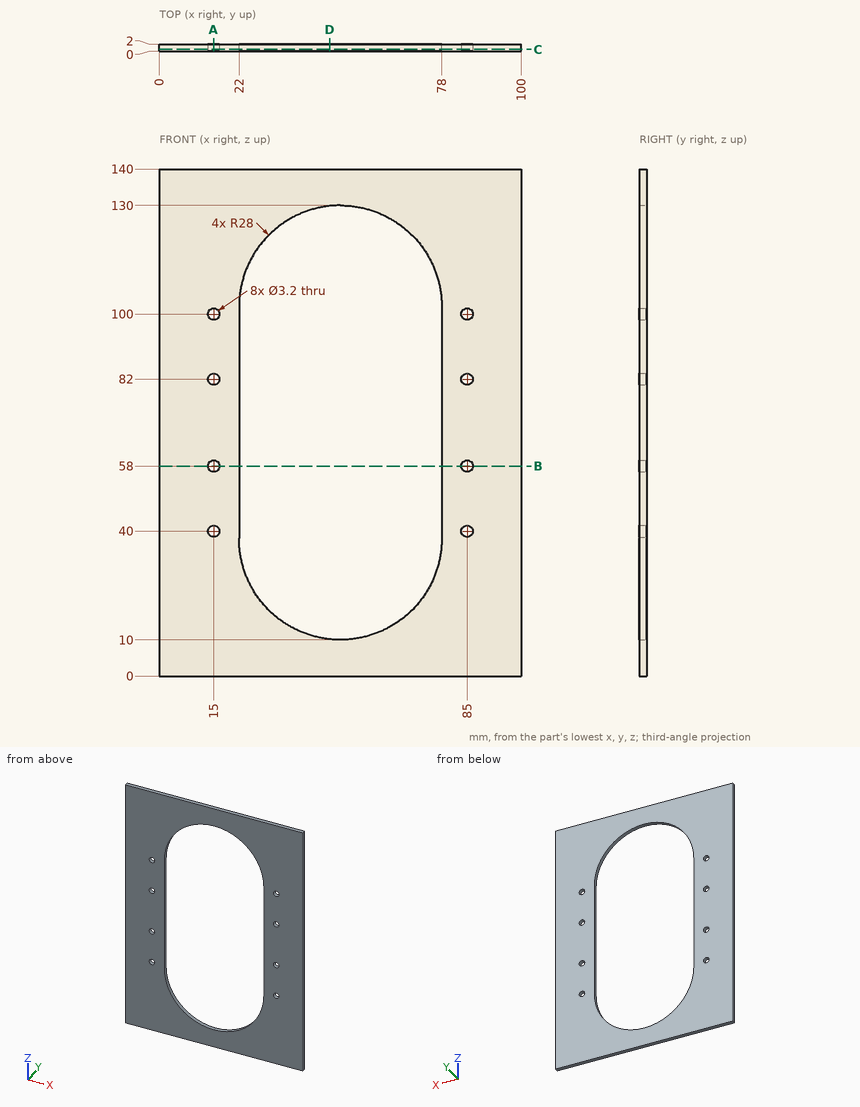
Drawing for the job (mm, zero at the part's lowest x, y, z). Give positions to 0.01 mm unless a question says otherwise; leave off trailing zeros. Loops run counter-clockwise (first coordinate to the right, second up) from the corner with the lowest first, then second, coordinate; pieces in that order, holes last.
Item 1: Slice it at C-C (y = 0.5). Give the number of separate pieces and of enclosed holes in the cut face, plus the area to 3 significant figures.
Check values:
separate pieces: 1
enclosed holes: 9
area: 7,890 mm2
Item 2: Slice it at A-A (x = 15). Write the cut outline in (y, z).
Check values:
outline: (0, 0) - (2, 0) - (2, 38.4) - (0, 38.4) - close; (0, 41.6) - (2, 41.6) - (2, 56.4) - (0, 56.4) - close; (0, 59.6) - (2, 59.6) - (2, 80.4) - (0, 80.4) - close; (0, 83.6) - (2, 83.6) - (2, 98.4) - (0, 98.4) - close; (0, 101.6) - (2, 101.6) - (2, 140) - (0, 140) - close
Item 3: Slice it at B-B (z = 58). Write the cut outline in (x, y).
Check values:
outline: (0, 0) - (13.4, 0) - (13.4, 2) - (0, 2) - close; (16.6, 0) - (22, 0) - (22, 2) - (16.6, 2) - close; (78, 0) - (83.4, 0) - (83.4, 2) - (78, 2) - close; (86.6, 0) - (100, 0) - (100, 2) - (86.6, 2) - close
Item 4: Slice it at D-D (x = 47). Write the cut outline in (y, z).
Check values:
outline: (0, 0) - (2, 0) - (2, 10.16) - (0, 10.16) - close; (0, 129.84) - (2, 129.84) - (2, 140) - (0, 140) - close
Item 5: Drill centre lines: line 1 along X through (y, z) = (1.1, 100); line 2 along Z through (x, y) = (85, 0.95); line 3 along X through (y, z) = (0.9, 102). Where is each one in solid material? Low to high.
Check values:
line 1: x = 0 to 13.4, 16.6 to 22, 78 to 83.4, 86.6 to 100
line 2: z = 0 to 38.4, 41.6 to 56.4, 59.6 to 80.4, 83.6 to 98.4, 101.6 to 140
line 3: x = 0 to 22, 78 to 100
